The listing builds one solid part. Answer for the finished solid, in the listing's coordinates (mm). A direction names the side the tool comes from. Give positions to 0.01 mm unless a question says otherwise; leave off trailing zeros. Order: outer loops, then holes, each group sorted by start corner. A loop starts at its lowest first (then second) coordinate and runs counter-clockwise, first axis right, second up. Notation, with made-up numbers: (81, -29) - (90, -29) arc R26 ccw to (90, -8) - close; hole circle Ø4 at (-14.5, 32.5). An arc over 180 degrees is marked (long way). Answer in a Markdown table with one row per item. Add a question column.
```python
from build123d import *

# Parameters (mm, degrees)
F0_R     = 9.5
F1_DEPTH = 38
F2_R     = 2.5
F3_R     = 9
F4_DEPTH = 6.64
F5_R     = 8.5
F6_DEPTH = 28.4


with BuildPart() as f1:
    # F0 (on Top) → F1 (new body)
    with BuildSketch(Plane.XY):
        Circle(F0_R)
    extrude(amount=F1_DEPTH)

    # F2
    f2_edges = [f1.edges().sort_by_distance(p)[0] for p in [
        (-9.5, 0, 38),
    ]]
    fillet(f2_edges, radius=F2_R)

    # F3 (on face) → F4 (cut)
    with BuildSketch(Plane(origin=(0, 0, 0), x_dir=(1, 0, 0), z_dir=(0, 0, -1))):
        Circle(F3_R)
    extrude(amount=-F4_DEPTH, mode=Mode.SUBTRACT)

    # F5 (on face) → F6 (cut)
    with BuildSketch(Plane(origin=(0, 0, 6.64), x_dir=(1, 0, 0), z_dir=(0, 0, -1))):
        Circle(F5_R)
    extrude(amount=-F6_DEPTH, mode=Mode.SUBTRACT)


solid = f1.part
```
(1) Find section D-D, the plane z = 3. Write down the section's boundary in (x, y), plus the area to 3 significant figures.
(2) Find section A-A, the plane y = 0. Write down the section's boundary in (x, z).
(3) For faces 1 (the face through (-6, -7, 0)), 2 (the face through (-1.172, -8.923, 3.274)), determine the directions among +Z, -Z, +X, -X, +Y, -Y from which every point of the face is accessible in a straight line to the end or side of a thin tool.
(4) Find section C-C, the plane z = 33. Write down the section's boundary in (x, y).
(5) Each of these flat-tipped pins is pushed along its axis until it touches: P1, Ø4, axis at x = 3, z = 20, coming from the +Y side; P2, Ø3, axis at x = -4.5, z = 18.5, coming from the +Y side; P3, Ø6, axis at x = -2, y = 1, coming from the -Z side. Where does it stop, or does it pass through?
(6) Straight lines are drawn through the part: line 1 (Y direction, x = 0, z = 3.25); line 2 (Y direction, x = 0, z = 22); line 3 (Z direction, x = 3.75, y = -5). For each, find the intervals that lie inside material, in ascending order.
(7) The mould has two halves that part along X. Classify faces 3 (the face through (0, 0, 38)), 4 (the face through (8, 3.3, 6.64)), 5 (the face through (4.38, -8.43, 17.5)): +X half, -X half, draft (parallel to the pull), parting line (faces both ways), or undercut.
Answer key:
| question | item | result |
|---|---|---|
| 1 | outline | circle Ø19 at (0, 0); hole circle Ø18 at (0, 0) |
| 1 | area | 29.1 mm² |
| 2 | outline | (-9.5, 0) - (-9, 0) - (-9, 6.64) - (-8.5, 6.64) - (-8.5, 35.04) - (8.5, 35.04) - (8.5, 6.64) - (9, 6.64) - (9, 0) - (9.5, 0) - (9.5, 35.5) arc R2.5 ccw to (7, 38) - (-7, 38) arc R2.5 ccw to (-9.5, 35.5) - close |
| 3 | face 1 | -Z, +X, -X, +Y, -Y |
| 3 | face 2 | -Z |
| 4 | outline | circle Ø19 at (0, 0); hole circle Ø17 at (0, 0) |
| 5 | P1 | y = 9.45 |
| 5 | P2 | y = 9.01 |
| 5 | P3 | z = 35.04 |
| 6 | line 1 | -9.5 to -9, 9 to 9.5 |
| 6 | line 2 | -9.5 to -8.5, 8.5 to 9.5 |
| 6 | line 3 | 35.04 to 38 |
| 7 | face 3 | draft |
| 7 | face 4 | undercut |
| 7 | face 5 | parting line |
